Design review of the part built by this model. Coordinates are the model's own, in mm. Coordinates: 2 decimals unless noted, no trailing zeros. Order: outer loops, then holes, each group sorted by start corner. A loop starts at its lowest first (then second) coordinate and runs counter-clockwise, first axis right, second up. Notation, with made-up numbers: (31, 45) -> (45, 45) arc R19 cw to (45, 73) -> close; hole circle Ø2 at (79, 20.5). An arc over 180 degrees is marked (long way). Use a Markdown table: item, result. Add a question column.
Q1. Add section A-A (z = 15). State the section outline as (x, y) points.
Q2. Add section C-C (y = -8.5). State the section outline as (x, z) points (3 decimals), then the cut area to 3 significant figures.
Q3. Add section D-D (x = -77.5). State the section outline as (y, z) points.
Q4. Insertion check: pin 1 (3 mm diameter, centred on y = -3.5, z = -5, fed in from -X); pin 2 (12.5 mm diameter, centred on x = -113.76, z = 12.02, fed in from +Y); pin 3 (1.5 mm diameter, centred on x = -17.5, y = -5.5, fed in from -Z); pin 4 (5 mm diameter, centred on x = 107, y = -8.5, fed in from +Z). Each pin has a flat end and moves straight along its axis. Give the tip position at first contact, or say it passes through.
Q5. Wall thickness on probe 1 along X at (y, z) = (-5.5, 5); probe 2 along X at (y, z) = (-0.25, -60); probe 3 along X at (y, z) = (-3.5, -32.5): over which ranges is each line inside the solid? List them lowest first.
Q6. The part is to be moulded in two halves that separate along Z. For faces 1 (the face through (4.02, -4.93, -30.06)), 2 (the face through (59.73, -4.93, -31.45)), 3 (the face through (-122.09, -4.93, 5.63)), 4 (the face through (51.786, -5, -52)), say which applies: pulls with the +Z half, pulls with the -Z half, needs draft (parallel to the pull), parting line crosses it, or undercut.
Q7. Add section B-B (z = -26.5). State the section outline as (x, y) points, then the cut area to 3 significant figures.
from build123d import *

# Parameters (mm, degrees)
F0_R     = 10.5
F1_DEPTH = 10


# Not quite as in the source:
# - ends of sketch curves that miss each other by under 0.0002 mm in the source are joined


with BuildPart() as f1:
    # F0 (on Front) → F1 (new body)
    with BuildSketch(Plane.XZ):
        with BuildLine():
            Line((-98.7553787733, 42.4647671212), (-118.7477670626, 42.4546280338))
            ThreePointArc((-118.7477670626, 42.4546280338), (-129.3548271656, 38.0531599477), (-133.7401521369, 27.4394155453))
            Line((-133.7401521369, 27.4394155453), (-133.71447629, 2.1254326641))
            Line((-133.71447629, 2.1254326641), (-133.71447629, -9.4965361613))
            ThreePointArc((-133.71447629, -9.4965361613), (-110.2994737436, -17.0606664942), (-85.71447629, -16.0328960194))
            ThreePointArc((-85.71447629, -16.0328960194), (-70.8573251513, -24.4500205619), (-55.2321770125, -31.3375216442))
            Line((-55.2321770125, -31.3375216442), (-39.21447629, -31.8745673359))
            Line((-39.21447629, -31.8745673359), (-39.1571401322, -35.2863552357))
            Line((-39.1571401322, -35.2863552357), (-39.0604409149, -67.8742687524))
            Line((-39.0604409149, -67.8742687524), (51.78552371, -67.7394838983))
            Line((51.78552371, -67.7394838983), (51.78552371, -35.1514269125))
            Line((51.78552371, -35.1514269125), (51.8327357464, -31.7394838983))
            Line((51.8327357464, -31.7394838983), (67.8487723641, -31.1549109155))
            ThreePointArc((67.8487723641, -31.1549109155), (83.4534142883, -24.2210753293), (98.28552371, -15.7599019106))
            ThreePointArc((98.28552371, -15.7599019106), (122.8456433746, -16.920758379), (146.28552371, -9.4965361613))
            Line((146.28552371, -9.4965361613), (146.28552371, 2.1254326641))
            Line((146.28552371, 2.1254326641), (146.1826080128, 27.4394155453))
            ThreePointArc((146.1826080128, 27.4394155453), (141.7598617434, 38.0144245463), (131.1604712744, 42.378416024))
            Line((131.1604712744, 42.378416024), (111.8151785594, 42.3497066713))
            ThreePointArc((111.8151785594, 42.3497066713), (6.5106579482, 7.1928164678), (-98.7553787733, 42.4647671212))
        make_face()
        with Locations((6.2913256733, -19.8069641195)):
            Circle(F0_R, mode=Mode.SUBTRACT)
        with Locations((-113.7560071881, 12.015007423)):
            Circle(F0_R, mode=Mode.SUBTRACT)
        with Locations((126.2437040296, 12.371086267)):
            Circle(F0_R, mode=Mode.SUBTRACT)
    extrude(amount=F1_DEPTH)


solid = f1.part
Established:
| question | item | result |
|---|---|---|
| 1 | outline | (-133.73, -10) -> (-123.82, -10) -> (-123.82, 0) -> (-133.73, 0) -> close; (-103.69, -10) -> (-45.08, -10) -> (-45.08, 0) -> (-103.69, 0) -> close; (58.29, -10) -> (116.08, -10) -> (116.08, 0) -> (58.29, 0) -> close; (136.41, -10) -> (146.23, -10) -> (146.23, 0) -> (136.41, 0) -> close |
| 2 | outline | (-133.74, 27.439) -> (-133.714, 2.125) -> (-133.714, -9.497) arc R69.826 ccw to (-85.714, -16.033) arc R170.357 ccw to (-55.232, -31.338) -> (-39.214, -31.875) -> (-39.157, -35.286) -> (-39.06, -67.874) -> (51.786, -67.739) -> (51.786, -35.151) -> (51.833, -31.739) -> (67.849, -31.155) arc R170.357 ccw to (98.286, -15.76) arc R69.826 ccw to (146.286, -9.497) -> (146.286, 2.125) -> (146.183, 27.439) arc R15 ccw to (131.16, 42.378) -> (111.815, 42.35) arc R175 cw to (-98.755, 42.465) -> (-118.748, 42.455) arc R15 ccw to start; hole circle Ø21 at (-113.756, 12.015); hole circle Ø21 at (6.291, -19.807); hole circle Ø21 at (126.244, 12.371) |
| 2 | area | 15,800 mm^2 |
| 3 | outline | (-10, -20.93) -> (0, -20.93) -> (0, 28.73) -> (-10, 28.73) -> close |
| 4 | pin 1 | x = -133.71 |
| 4 | pin 2 | through |
| 4 | pin 3 | z = -67.84 |
| 4 | pin 4 | z = 40.64 |
| 5 | probe 1 | -133.72 to -121.57, -105.94 to 118.77, 133.72 to 146.27 |
| 5 | probe 2 | -39.08 to 51.79 |
| 5 | probe 3 | -39.2 to 51.82 |
| 6 | face 1 | undercut |
| 6 | face 2 | pulls with the -Z half |
| 6 | face 3 | undercut |
| 6 | face 4 | needs draft |
| 7 | outline | (-66.63, -10) -> (-1.8, -10) -> (-1.8, 0) -> (-66.63, 0) -> close; (14.38, -10) -> (78.77, -10) -> (78.77, 0) -> (14.38, 0) -> close |
| 7 | area | 1,290 mm^2 |
